Read the model definition and answer for the solid it produces. Units are mm, in the model's axes. A direction names the side the tool comes from. Coordinates: 2 decimals unless noted, no trailing zeros. Loops run counter-clockwise (first coordinate to the right, second up) from the corner with the lowest first, then second, coordinate; pieces in that order, holes last. Notation, with made-up numbers: (27.25, 86.5) -> (61.25, 86.5) arc R22 cw to (61.25, 100.5) -> close; hole circle Ø1 at (26, -36). An arc over 180 degrees is marked (long way). Answer as a JSON object with one key per item and string values. Group by question number.
Q1. For faces 1 (the cylindrical face through (64.8, 3.22, -112.07)), 2 (the cylindrical face through (-142.76, 3.22, 142.36)), determine the directions among +Z, -Z, +X, -X, +Y, -Y from which every point of the face is accessible in a straight line to the end or side of a thin tool.
Q2. The part is cut by section B-B on z = -111.9. Write down the section's boundary in (x, y).
Q3. The part is cut by section A-A on x = -15. Write down the section's boundary in (y, z).
Q4. The part is cut by section C-C on z = 110. Write down the section's boundary in (x, y).
Q5. Straight lines are drawn through the part: line 1 along X through (y, z) = (4, 111.9); line 2 along Z through (x, y) = (111, 1.25); line 3 along X through (y, z) = (5.25, -3). For each, find the intervals that lie inside material, in ascending order. Write a range as [from, to].
Q6. This flat-tipped pin is pushed along its axis until it touches: P1, Ø1.9, axis at x = -131.5, y = 2, coming from the +Z side. Where does it stop, or does it pass through?
Q7. The part is cut by section D-D on x = -111.9. Write down the section's boundary in (y, z), and give its area (3 significant figures).
Q8. Determine the mould class of faces 3 (the cylindrical face through (-142.76, 3.22, -142.36)), 4 (the cylindrical face through (126.38, 3.22, 96.1)), 5 (the cylindrical face through (142.36, 3.22, 142.76)), 6 (the flat face through (-2, 0, -2)) for opening direction X: released by +X, released by -X, zero draft, split by the parting line, or undercut.
from build123d import *

# Parameters (mm, degrees)
SKETCH1_W           = 300
SKETCH1_H           = 300
BOSS_EXTRUDE1_DEPTH = 6.35
SKETCH2_R           = 2.0828
SKETCH2_R_2         = 2.778125
SKETCH2_R_3         = 21.43125
SKETCH2_W           = 22.86
SKETCH2_H           = 63.5
CUT_EXTRUDE1_DEPTH  = 213.227054119
FILLET1_R           = 25.4


with BuildPart() as part:
    # Sketch1 → Boss-Extrude1 (new body)
    with BuildSketch(Plane(origin=(0, 0, 0), x_dir=(1, 0, 0), z_dir=(0, 1, 0))):
        Rectangle(SKETCH1_W, SKETCH1_H)
    extrude(amount=BOSS_EXTRUDE1_DEPTH)

    # Sketch2 → Cut-Extrude1 (cut, through all)
    with BuildSketch(Plane(origin=(0, 6.35, 0), x_dir=(1, 0, 0), z_dir=(0, 1, 0))):
        with Locations(Location((-87.138207153, 87.138207153, 0), (0, 0, 270))):
            Circle(SKETCH2_R)
        with Locations(Location((87.138207153, 87.138207153, 0), (0, 0, 90))):
            Circle(SKETCH2_R)
        with Locations(Location((87.138207153, -87.138207153, 0), (0, 0, 270))):
            Circle(SKETCH2_R)
        with Locations(Location((-87.138207153, -87.138207153, 0), (0, 0, 90))):
            Circle(SKETCH2_R)
        with Locations(Location((-141.6688, 61.1, 0), (0, 0, 270))):
            Circle(SKETCH2_R)
        with Locations(Location((-141.6688, -61.1, 0), (0, 0, 270))):
            Circle(SKETCH2_R)
        with Locations(Location((-76.2, -141.6688, 0), (0, 0, 270))):
            Circle(SKETCH2_R)
        with Locations(Location((76.2, -141.6688, 0), (0, 0, 270))):
            Circle(SKETCH2_R)
        with Locations(Location((0, -141.6688, 0), (0, 0, 270))):
            Circle(SKETCH2_R)
        with Locations(Location((-76.2, 141.6688, 0), (0, 0, 270))):
            Circle(SKETCH2_R)
        with Locations(Location((76.2, 141.6688, 0), (0, 0, 270))):
            Circle(SKETCH2_R)
        with Locations(Location((141.6688, 61.1, 0), (0, 0, 270))):
            Circle(SKETCH2_R)
        with Locations(Location((141.6688, -61.1, 0), (0, 0, 270))):
            Circle(SKETCH2_R)
        with Locations(Location((-139.6622, 40.4492, 0), (0, 0, 270))):
            Circle(SKETCH2_R)
        with Locations(Location((-124.7778, 40.4492, 0), (0, 0, 270))):
            Circle(SKETCH2_R)
        with Locations(Location((-139.6622, -40.2212, 0), (0, 0, 270))):
            Circle(SKETCH2_R)
        with Locations(Location((-124.7778, -40.2212, 0), (0, 0, 270))):
            Circle(SKETCH2_R)
        with Locations(Location((124.7778, 40.4492, 0), (0, 0, 270))):
            Circle(SKETCH2_R)
        with Locations(Location((139.6622, 40.4492, 0), (0, 0, 270))):
            Circle(SKETCH2_R)
        with Locations(Location((124.7778, -40.2212, 0), (0, 0, 270))):
            Circle(SKETCH2_R)
        with Locations(Location((139.6622, -40.2212, 0), (0, 0, 270))):
            Circle(SKETCH2_R)
        with Locations(Location((-58.438333333, 26.439261833, 0), (0, 0, 270))):
            Circle(SKETCH2_R)
        with Locations(Location((-58.438333333, -26.211261833, 0), (0, 0, 270))):
            Circle(SKETCH2_R)
        with Locations(Location((58.438333333, 26.439261833, 0), (0, 0, 270))):
            Circle(SKETCH2_R)
        with Locations(Location((58.438333333, -26.211261833, 0), (0, 0, 270))):
            Circle(SKETCH2_R)
        with Locations(Location((-131.28002933, -91.994917364, 0), (0, 0, 270))):
            Circle(SKETCH2_R_2)
        with Locations(Location((-111.9, -111.9, 0), (0, 0, 270))):
            Circle(SKETCH2_R_3)
        with Locations(Location((-92.51997067, -131.805082636, 0), (0, 0, 90))):
            Circle(SKETCH2_R_2)
        with Locations(Location((91.994917364, -131.28002933, 0), (0, 0, 270))):
            Circle(SKETCH2_R_2)
        with Locations(Location((111.9, -111.9, 0), (0, 0, 270))):
            Circle(SKETCH2_R_3)
        with Locations(Location((131.805082636, -92.51997067, 0), (0, 0, 90))):
            Circle(SKETCH2_R_2)
        with Locations(Location((91.575239032, 130.839428269, 0), (0, 0, 270))):
            Circle(SKETCH2_R_2)
        with Locations(Location((111.9, 111.9, 0), (0, 0, 270))):
            Circle(SKETCH2_R_3)
        with Locations(Location((132.224760968, 92.960571731, 0), (0, 0, 90))):
            Circle(SKETCH2_R_2)
        with Locations(Location((-130.839428269, 91.575239032, 0), (0, 0, 270))):
            Circle(SKETCH2_R_2)
        with Locations(Location((-111.9, 111.9, 0), (0, 0, 270))):
            Circle(SKETCH2_R_3)
        with Locations(Location((-92.960571731, 132.224760968, 0), (0, 0, 90))):
            Circle(SKETCH2_R_2)
        with BuildLine():
            Line((-57.15, 119.55), (57.15, 119.55))
            ThreePointArc((57.15, 119.55), (64.8, 111.9), (57.15, 104.25))
            Line((57.15, 104.25), (-57.15, 104.25))
            ThreePointArc((-57.15, 104.25), (-64.8, 111.9), (-57.15, 119.55))
        make_face()
        with Locations((132.22, 0)):
            Rectangle(SKETCH2_W, SKETCH2_H)
        with Locations((-132.219999948, 0)):
            Rectangle(SKETCH2_W, SKETCH2_H)
    extrude(amount=-CUT_EXTRUDE1_DEPTH, mode=Mode.SUBTRACT)

    # Fillet1
    fillet1_edges = [part.edges().sort_by_distance(p)[0] for p in [
        (150, 3.175, 150),
        (-150, 3.175, 150),
        (-150, 3.175, -150),
        (150, 3.175, -150),
    ]]
    fillet(fillet1_edges, radius=FILLET1_R)


solid = part.part
Final values:
{
 "1": {"face 1": "+Y, -Y", "face 2": "+Z, -X, +Y, -Y"},
 "2": {"outline": "(-150, 0) -> (-133.33, 0) -> (-133.33, 6.35) -> (-150, 6.35) -> close; (-90.47, 0) -> (-64.8, 0) -> (-64.8, 6.35) -> (-90.47, 6.35) -> close; (64.8, 0) -> (90.47, 0) -> (90.47, 6.35) -> (64.8, 6.35) -> close; (133.33, 0) -> (150, 0) -> (150, 6.35) -> (133.33, 6.35) -> close"},
 "3": {"outline": "(0, -150) -> (6.35, -150) -> (6.35, -119.55) -> (0, -119.55) -> close; (0, -104.25) -> (6.35, -104.25) -> (6.35, 150) -> (0, 150) -> close"},
 "4": {"outline": "(-150, 0) -> (-133.25, 0) -> (-133.25, 6.35) -> (-150, 6.35) -> close; (-90.55, 0) -> (90.55, 0) -> (90.55, 6.35) -> (-90.55, 6.35) -> close; (133.25, 0) -> (150, 0) -> (150, 6.35) -> (133.25, 6.35) -> close"},
 "5": {"line 1": "x = [-150, -133.33], [-90.47, 90.47], [133.33, 150]", "line 2": "z = [-150, -133.31], [-90.49, 90.49], [133.31, 150]", "line 3": "x = [-150, -143.65], [-120.79, 120.79], [143.65, 150]"},
 "6": {"P1": "stops at z = 149.29"},
 "7": {"outline": "(0, -150) -> (6.35, -150) -> (6.35, -133.33) -> (0, -133.33) -> close; (0, -90.47) -> (6.35, -90.47) -> (6.35, 90.47) -> (0, 90.47) -> close; (0, 133.33) -> (6.35, 133.33) -> (6.35, 150) -> (0, 150) -> close", "area": "1,360 mm2"},
 "8": {"face 3": "released by -X", "face 4": "undercut", "face 5": "released by +X", "face 6": "zero draft"}
}
